Part print with two shaded views. Sizes in mm from the minimum x, y, z corner. Round coordinates to 2 decimals unless told otherwise and drop trailing zeros. Order: outer loops, then holes, each group sorted by start corner. A loop starts at its lowest first (then second) coordinate and runs counter-clockwise, first axis right, second up. Notation, with made-up numbers: (39.5, 83) -> (74.5, 83) arc R22 ccw to (74.5, 95) -> close; hole circle Ø10 at (14.25, 46.25). An arc over 180 degrees is marked (long way). Use a Markdown table: item, result. Add a question column.
Item 1: Slice it at B-B, the plane x = 3. Give the cut face in (y, z).
Item 2: Slice it at C-C, the plane y = 5. Give the cut face in (x, z), plus the area to 3 significant figures.
Item 3: Slice it at A-A, the plane z = 3. Give the cut face in (x, y).
Item 4: Pin check, flat tip, straight feed: pin 1 (1.5 mm diameter, centred on y = 7, z = 2, fed in from +X). Stop position of the tip, or through.
Item 5: Probe L1, parallel to Y at x = 4.95, z = 1.7; L2, parallel to X at y = 9.25, z = 2.9. List the from-to ranges inside material, lowest first.
Item 6: Slice it at D-D, the plane y = 1.75. Give the cut face in (x, z).
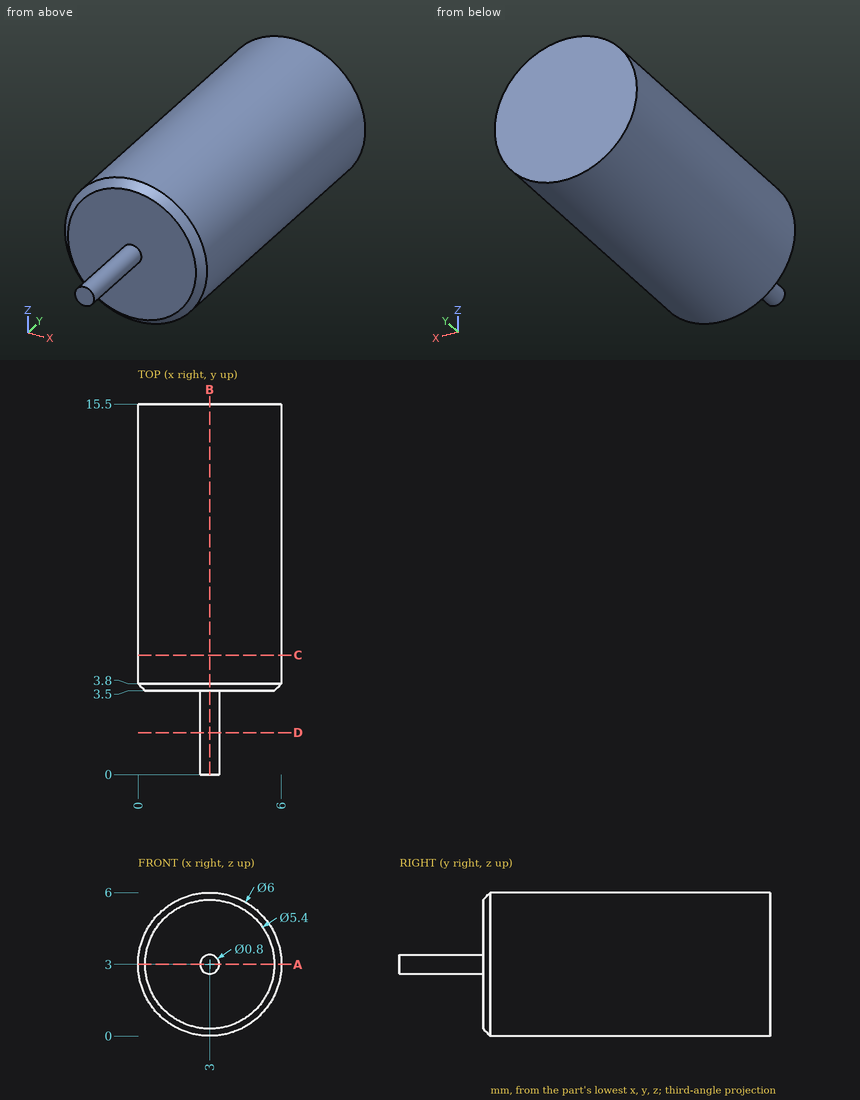
Check sheet entries:
| question | item | result |
|---|---|---|
| 1 | outline | (0, 2.6) -> (3.5, 2.6) -> (3.5, 0.3) -> (3.8, 0) -> (15.5, 0) -> (15.5, 6) -> (3.8, 6) -> (3.5, 5.7) -> (3.5, 3.4) -> (0, 3.4) -> close |
| 2 | outline | circle Ø6 at (3, 3) |
| 2 | area | 28.3 mm2 |
| 3 | outline | (0, 3.8) -> (0.3, 3.5) -> (2.6, 3.5) -> (2.6, 0) -> (3.4, 0) -> (3.4, 3.5) -> (5.7, 3.5) -> (6, 3.8) -> (6, 15.5) -> (0, 15.5) -> close |
| 4 | pin 1 | x = 5.99 |
| 5 | L1 | 3.5 to 15.5 |
| 5 | L2 | 0 to 6 |
| 6 | outline | circle Ø0.8 at (3, 3) |
